from build123d import *

# Parameters (mm, degrees)
F0_W     = 457.2
F0_H     = 254
F1_DEPTH = 254
F2_W     = 25.4
F2_H     = 25.4
F3_DEPTH = 25.4
F4_R     = 279.4
F5_DEPTH = 203.2


with BuildPart() as f1:
    # F0 (on Front) → F1 (new body)
    with BuildSketch(Plane.XZ):
        with Locations((228.6, 127)):
            Rectangle(F0_W, F0_H)
    extrude(amount=F1_DEPTH)

    # F2 (on face) → F3 (join)
    with BuildSketch(Plane.YZ.offset(457.2)):
        with Locations((-127, 127)):
            Rectangle(F2_W, F2_H)
    extrude(amount=F3_DEPTH)

    # F4 (on face) → F5 (join)
    with BuildSketch(Plane.YZ.offset(482.6)):
        with Locations((-127, 127)):
            Circle(F4_R)
    extrude(amount=F5_DEPTH)


solid = f1.part
The listing builds one solid part. Answer for the finished solid, in the listing's coordinates (mm). A direction names the side the tool comes from. Coordinates: 2 decimals unless noted, no trailing zeros. Order: outer loops, then holes, each group sorted by start corner. A loop starts at its lowest first (then second) coordinate and runs counter-clockwise, first axis right, second up.
Q1. A cutting plane is placed at A-A, the plane z = 84.5. Write down the section's boundary in (x, y).
Q2. Which of the six approach directions +Z, -Z, +X, -X, +Y, -Y give full straight-line access (tool end or side, diameter ignored) to faces 4 (the face through (225, 0, 129)), 5 (the face through (225, -125, 0)), 6 (the face through (470, -127, 114.3)), 7 (the face through (225, -125, 254)), 8 (the face through (470, -139.7, 127))?
Q3. A cutting plane is placed at C-C, the plane y = -210. Write down the section's boundary in (x, z), and give its area (3 significant figures).
Q4. For a pull along X with two mould halves and no side action, classify faces 1 (the face through (470, -127, 139.7)), 2 (the face through (685.8, -131, 131)), 3 (the face through (225, -254, 129)) as pulls with the +X half, pulls with the -X half, needs draft (parallel to the pull), parting line crosses it, or undercut.
Q5. A cutting plane is placed at D-D, the plane x = 447. Write down the section's boundary in (y, z), and give its area (3 significant figures).
Q6. Given P1, Ø12, axis at x = 538, z = 228.5, coming from the -Y side; P2, Ø10, axis at x = 149, y = -34.5, coming from the -Z side; P3, Ø12.5, axis at x = 466, z = 124.5, coming from the -Y side, each flat-ended and moving along its own axis, determine where each tip first touches the part or whether it passes through.
Q7. Consider line 1 (X direction, y = -235, z = 214.5); line 2 (Y direction, x = 148, z = 105.5); line 3 (X direction, y = -210, z = 337). Determine where each line is inside the solid, lowest interval first.
Q8. A cutting plane is placed at B-B, the plane y = -127. Write down the section's boundary in (x, z), and give its area (3 significant figures).
Answers follow:
1. outline: (0, -254) - (457.2, -254) - (457.2, 0) - (0, 0) - close; (482.6, -403.15) - (685.8, -403.15) - (685.8, 149.15) - (482.6, 149.15) - close
2. face 4: +Z, -Z, -X, +Y
2. face 5: -Z, -X, +Y, -Y
2. face 6: -Z, +Y, -Y
2. face 7: +Z, -X, +Y, -Y
2. face 8: +Z, -Z, -Y
3. outline: (0, 0) - (457.2, 0) - (457.2, 254) - (0, 254) - close; (482.6, -139.79) - (685.8, -139.79) - (685.8, 393.79) - (482.6, 393.79) - close
3. area: 225,000 mm2
4. face 1: undercut
4. face 2: pulls with the +X half
4. face 3: needs draft
5. outline: (-254, 0) - (0, 0) - (0, 254) - (-254, 254) - close
5. area: 64,500 mm2
6. P1: stops at y = -389.57
6. P2: stops at z = 0
6. P3: stops at y = -139.7
7. line 1: x = 0 to 457.2, 482.6 to 685.8
7. line 2: y = -254 to 0
7. line 3: x = 482.6 to 685.8
8. outline: (0, 0) - (457.2, 0) - (457.2, 114.3) - (482.6, 114.3) - (482.6, -152.4) - (685.8, -152.4) - (685.8, 406.4) - (482.6, 406.4) - (482.6, 139.7) - (457.2, 139.7) - (457.2, 254) - (0, 254) - close
8. area: 230,000 mm2
